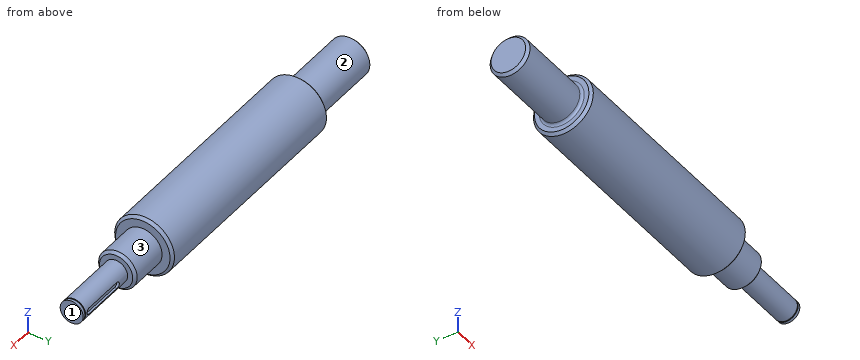
from build123d import *

# Parameters (mm, degrees)
CHAMFER1_SIZE      = 2.54
CHAMFER2_SIZE      = 2.54
FILLET1_R          = 2.54
CUT_EXTRUDE2_DEPTH = 2.5
SKETCH7_R          = 11
SKETCH7_R_2        = 10.35
CUT_EXTRUDE3_DEPTH = 1.1


with BuildPart() as part:
    # Sketch1 → Revolve1 (revolve)
    with BuildSketch(Plane.XY, mode=Mode.PRIVATE) as revolve1_sk:
        Polygon((-200, 0), (200, 0), (200, 11), (136.5, 11), (136.5, 18.415), (98.4, 18.415), (98.4, 28.575), (-123.8, 28.575), (-123.8, 19.05), (-200, 19.05), align=None)
    revolve(revolve1_sk.sketch.rotate(Axis((-1910.961105754, 0, 0), (1, 0, 0)), 90), axis=Axis((-1910.961105754, 0, 0), (1, 0, 0)))

    # Chamfer1
    chamfer1_edges = [part.edges().sort_by_distance(p)[0] for p in [
        (136.5, 0, -18.415),
        (98.4, 0, -28.575),
    ]]
    chamfer(chamfer1_edges, length=CHAMFER1_SIZE)

    # Chamfer2
    chamfer2_edges = [part.edges().sort_by_distance(p)[0] for p in [
        (-123.8, 0, -28.575),
        (-200, 0, -19.05),
    ]]
    chamfer(chamfer2_edges, length=CHAMFER2_SIZE)

    # Fillet1
    fillet1_edges = [part.edges().sort_by_distance(p)[0] for p in [
        (-123.8, 0, -19.05),
    ]]
    fillet(fillet1_edges, radius=FILLET1_R)

    # Sketch3 → Cut-Extrude2 (cut)
    with BuildSketch(Plane(origin=(0, 11, 0), x_dir=(1, 0, 0), z_dir=(0, 1, 0))):
        with BuildLine():
            Line((151.375, 3), (191.375, 3))
            ThreePointArc((191.375, 3), (194.375, 0), (191.375, -3))
            Line((191.375, -3), (151.375, -3))
            ThreePointArc((151.375, -3), (148.375, 0), (151.375, 3))
        make_face()
    extrude(amount=-CUT_EXTRUDE2_DEPTH, mode=Mode.SUBTRACT)

    # Sketch7 → Cut-Extrude3 (cut)
    with BuildSketch(Plane(origin=(196.49768, 0, 0), x_dir=(0, 0, -1), z_dir=(1, 0, 0))):
        with Locations(Location((0, 0, 0), (0, 0, 180))):
            Circle(SKETCH7_R)
        Circle(SKETCH7_R_2, mode=Mode.SUBTRACT)
    extrude(amount=CUT_EXTRUDE3_DEPTH, mode=Mode.SUBTRACT)


solid = part.part
Design review of the part built by this model. Coordinates are the model's own, in mm. Face numbers are marked on the shaded views. A direction names the side the tool comes from. Coordinates: 2 decimals unless noted, no trailing zeros. Loops run counter-clockwise (first coordinate to the right, second up) from the corner with the lowest first, then second, coordinate; pieces in that order, holes last. Notation, with made-up numbers: (22.5, 35.5) -> (38.5, 35.5) arc R13 cw to (38.5, 56.5) -> close; hole circle Ø8 at (-32.75, -33.5). An arc over 180 degrees is marked (long way). Use a Markdown table: item, result. Add a question column.
Item 1: Machinability: for the marked faces 1, 2 and 3, which of the approach directions +Z, -Z, +X, -X, +Y, -Y give a long, thin tool a straight path to every point of the face, cutting with its end or side? Answer none if there is none.
Item 2: We need section C-C, the plane x = 85.5. Write out the cut boundary in (y, z) (3 decimals), and give its area (3 significant figures).
Item 3: Wall thickness on L1, parallel to X at y = -23.5, z = -2; L2, parallel to Y at x = -59, z = 1; L3, parallel to Y at x = -173.5, z = 0.5: over which ranges is each line inside the solid? List them lowest first. Write a range as from..to.
Item 4: We need section D-D, the plane x = -171. Write out the cut boundary in (y, z), and give its area (3 significant figures).
Item 5: Clearance check with flat-ended pins moving along their axes: P1, Ø1.5, axis at x = 121, y = 6, coming from the -Z side; P2, Ø2.5, axis at x = 166.5, y = 9.5, coming from the -Z side; P3, Ø4, axis at y = 13.5, z = -21, coming from the -X side. State where each tip first meets the part, or that it passes through.
Item 6: We need section B-B, the plane x = 156. Write out the cut boundary in (y, z).
Numbers:
| question | item | result |
|---|---|---|
| 1 | face 1 | +Z, -Z, +X, +Y, -Y |
| 1 | face 2 | -X |
| 1 | face 3 | +X |
| 2 | outline | circle Ø57.15 at (0, 0) |
| 2 | area | 2,570 mm^2 |
| 3 | L1 | x = -123.8..98.4 |
| 3 | L2 | y = -28.56..28.56 |
| 3 | L3 | y = -19.04..19.04 |
| 4 | outline | circle Ø38.1 at (0, 0) |
| 4 | area | 1,140 mm^2 |
| 5 | P1 | stops at z = -17.65 |
| 5 | P2 | stops at z = -7.28 |
| 5 | P3 | stops at x = -123.8 |
| 6 | outline | (8.5, -3) -> (8.5, 3) -> (10.58, 3) arc R11 ccw (long way) to (10.58, -3) -> close |
